Geometry: see drawing. Coordinates: mm, zero at the bounding-box minimum. A direction names the side the tool comes from. Give positions to 0.01 mm unless a question says otherwise; leave off trailing zeros. Write each loop counter-clockwise with the first axis right and the second up, starting at its lowest first coordinate (ties: lowest second). Pieces come first, ordered by that corner, then holes. Notation, with made-up numbers: (64.5, 73) - (98.5, 73) arc R19 cw to (98.5, 109) - close; hole circle Ø1 at (-14, -38.5). An arc over 180 degrees is marked (long way). One line per question, with ' | ' between items. Start each with the question number.
(1) Pin query (flat end, axial travel): pin 1 (6 mm diameter, centred on x = 24, y = 2, fed in from +Z); pin 2 (1.2 mm diameter, centred on x = 2, y = 9, fed in from -Z); pin 3 (4.5 mm diameter, centred on x = 1.5, y = 8, fed in from +Z); pin 4 (1.2 mm diameter, centred on x = 2, y = 6, fed in from +Z). Return the tip coordinate at first contact, or that it passes through.
(2) Access query for the marked faces 1, 2, 3, 4 and 5. Directions: +Z, -Z, +X, -X, +Y, -Y. A direction counts if a zero-diameter tool reaches every point of the face in a straight line with its end or side. Return the directions, or none.
(3) Section B-B, the plane x = 14. Return loops of the section in (y, z).
(4) Section A-A, the plane x = 28. Return loops of the section in (y, z), plus the area to 3 significant figures.
(5) Section C-C, the plane z = 21.75. Return loops of the section in (x, y).
(6) Section D-D, the plane y = 10.5. Return loops of the section in (x, z), plus the area to 3 significant figures.
(7) Ray query, line 1 (Y direction, x = 28, z = 10.65); line 2 (Z direction, x = 8.5, y = 9); line 3 (Z direction, x = 2, y = 4.75). Return the intervals inside material, ascending. Write a range as [from, to].
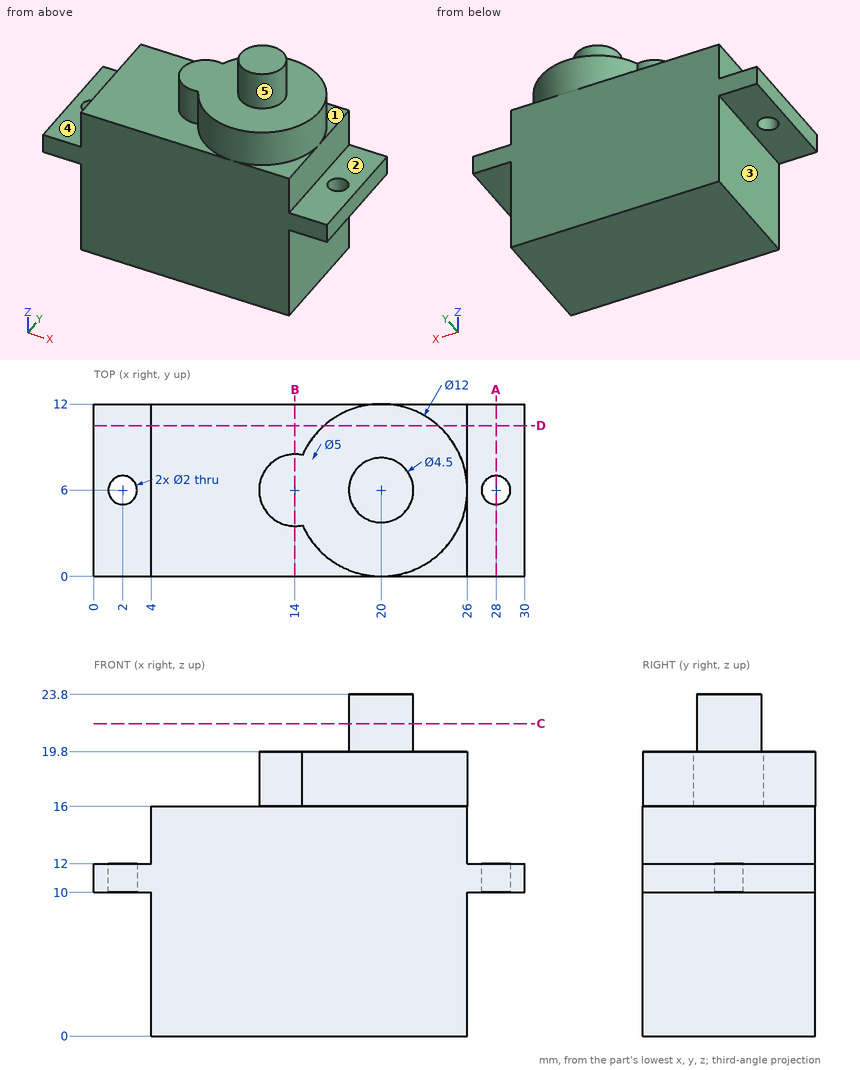
Check sheet entries:
1) pin 1: z = 19.8 | pin 2: z = 10 | pin 3: z = 12 | pin 4: through
2) face 1: +Z, +X, +Y | face 2: +Z, +X, +Y, -Y | face 3: -Z, -X, +Y, -Y | face 4: +Z, -X, +Y, -Y | face 5: +Z
3) outline: (0, 0) - (12, 0) - (12, 16) - (8.5, 16) - (8.5, 19.8) - (3.5, 19.8) - (3.5, 16) - (0, 16) - close
4) outline: (0, 10) - (5, 10) - (5, 12) - (0, 12) - close; (7, 10) - (12, 10) - (12, 12) - (7, 12) - close | area: 20.0 mm²
5) outline: circle Ø4.5 at (20, 6)
6) outline: (0, 10) - (4, 10) - (4, 0) - (26, 0) - (26, 10) - (30, 10) - (30, 12) - (26, 12) - (26, 16) - (23.97, 16) - (23.97, 19.8) - (16.03, 19.8) - (16.03, 16) - (4, 16) - (4, 12) - (0, 12) - close | area: 398 mm²
7) line 1: [0, 5], [7, 12] | line 2: [0, 16] | line 3: [10, 12]
